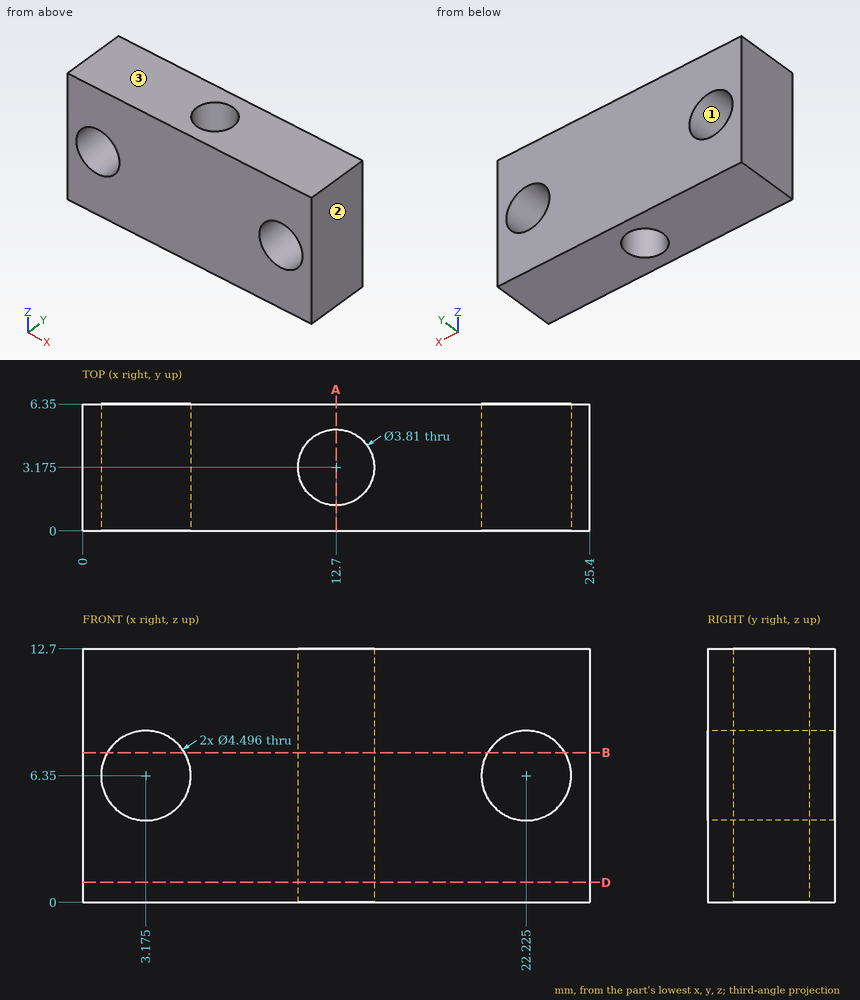
Job drawing, mm, ordinate dimensions from the low corner. One solid piece. Round coordinates to 2 decimals unless told otherwise and drop trailing zeros. Write each loop counter-clockwise with the first axis right and the second up, starting at its lowest first coordinate (ties: lowest second). Pieces come first, ordered by that corner, then holes.
1) Drill centre lines: probe 1 along Y at (x, z) = (12.7, 3); probe 2 along Z at (x, y) = (3.25, 1.5); probe 3 along Z at (x, y) = (1.25, 1.25). Where is each one in solid material? Low to high.
2) Band-saw the part on B-B, the plane z = 7.5. Give the number of separate pieces and of enclosed holes in the cut face, and give its area (3 significant figures).
3) Mould opens along Z. For the marked faces 1, 2 and 3 say: +Z half, -Z half, draft (parallel to the pull), parting line (faces both ways), or undercut.
4) Pin check, flat tip, straight feed: pin 1 (2.5 mm diameter, centred on x = 22.225, z = 6.35, fed in from +Y). Stop position of the tip, or through.
5) Band-saw the part on D-D, the plane z = 1. List the corners of the cut face in (x, y) (3 decimals).
6) Band-saw the part on A-A, the plane x = 12.7. List the corners of the cut face in (y, z).
Ans:
1. probe 1: y = 0 to 1.27, 5.08 to 6.35
1. probe 2: z = 0 to 4.1, 8.6 to 12.7
1. probe 3: z = 0 to 5.19, 7.51 to 12.7
2. separate pieces: 3
2. enclosed holes: 1
2. area: 101 mm2
3. face 1: undercut
3. face 2: draft
3. face 3: +Z half
4. pin 1: passes through
5. outline: (0, 0) - (25.4, 0) - (25.4, 6.35) - (0, 6.35) - close; hole circle Ø3.81 at (12.7, 3.175)
6. outline: (0, 0) - (1.27, 0) - (1.27, 12.7) - (0, 12.7) - close; (5.08, 0) - (6.35, 0) - (6.35, 12.7) - (5.08, 12.7) - close
